```python
from build123d import *

# Parameters (mm, degrees)
SKETCH1_R               = 50.8
BOSS_EXTRUDE1_DEPTH     = 2.54
BOSS_EXTRUDE2_DEPTH     = 10.16
FILLET1_R               = 1.27
CUT_EXTRUDE1_DEPTH      = 113.048264746
CUT_EXTRUDE1_DEPTH_BACK = 113.048264746
SKETCH3_R               = 2.54
SKETCH5_R               = 1.27
CUT_EXTRUDE2_DEPTH      = 73.556912988


# Read off the part's stored shape, not the designer's step: Boss-Extrude2
with BuildPart() as part:
    # Sketch1 → Boss-Extrude1 (new body)
    with BuildSketch(Plane(origin=(0, 0, 0), x_dir=(1, 0, 0), z_dir=(0, 1, 0))):
        with Locations(Location((0, 0, 0), (0, 0, 270))):
            Circle(SKETCH1_R)
    extrude(amount=BOSS_EXTRUDE1_DEPTH)


with BuildPart() as boss_extrude2_tool:
    # Boss-Extrude2 outline → Boss-Extrude2 (new body)
    with BuildSketch(Plane(origin=(0, 2.54, 0), x_dir=(1, 0, 0), z_dir=(0, 1, 0))):
        with BuildLine():
            Line((-5.08, -48.26), (-5.08, -50.545361805))
            add(Edge.make_bspline(
                [(5.08, -50.545361805), (0, -51.054638195), (-5.08, -50.545361805)],
                knots=[0, 0, 0, 1, 1, 1], degree=2))
            Line((5.08, -50.545361805), (5.08, -48.26))
            Line((5.08, -48.26), (-5.08, -48.26))
        make_face()
        with BuildLine():
            Line((5.08, 48.26), (5.08, 50.545361805))
            add(Edge.make_bspline(
                [(-5.08, 50.545361805), (0, 51.054638195), (5.08, 50.545361805)],
                knots=[0, 0, 0, 1, 1, 1], degree=2))
            Line((-5.08, 50.545361805), (-5.08, 48.26))
            Line((-5.08, 48.26), (5.08, 48.26))
        make_face()
    extrude(amount=BOSS_EXTRUDE2_DEPTH)


with BuildPart() as part_1:
    add(part.part)


with BuildPart() as part_2:
    # Boss-Extrude2: joined with boss_extrude2_tool
    add(part_1.part.fuse(boss_extrude2_tool.part, tol=0.00001))

    # Fillet1
    # the kernel refuses this fillet: 1.27 mm, written as the material it adds along each edge
    with BuildSketch(Plane(origin=(-5.08, 2.54, -48.26), x_dir=(0, 0, 1), z_dir=(1, 0, 0)), Plane(origin=(5.08, 2.54, 48.26), x_dir=(0, 0, -1), z_dir=(-1, 0, 0))) as fillet1_piece_1:
        with BuildLine():
            CenterArc((FILLET1_R, -FILLET1_R), FILLET1_R, 90, 90)
            Line((0, -FILLET1_R), (0, 0))
            Line((0, 0), (FILLET1_R, 0))
        make_face()
    extrude(amount=10.16)
    with BuildSketch(Plane(origin=(5.08, 2.54, -48.26), x_dir=(1, 0, 0), z_dir=(0, 0, -1))) as fillet1_piece_2_section:
        with BuildLine():
            CenterArc((FILLET1_R, -FILLET1_R), FILLET1_R, 90, 90)
            Line((0, -FILLET1_R), (0, 0))
            Line((0, 0), (FILLET1_R, 0))
        make_face()
    fillet1_piece_2 = extrude(amount=5.460361805, mode=Mode.PRIVATE)
    fillet1_piece_2 = fillet1_piece_2 & Plane(origin=(0, 2.829642474, 0), x_dir=(0, 0, 1), z_dir=(0, -1, 0)) * Cylinder(50.8, 17, mode=Mode.PRIVATE)
    add(fillet1_piece_2)
    with BuildSketch(Plane(origin=(5.08, 2.54, 53.720361805), x_dir=(1, 0, 0), z_dir=(0, 0, -1))) as fillet1_piece_3_section:
        with BuildLine():
            CenterArc((FILLET1_R, -FILLET1_R), FILLET1_R, 90, 90)
            Line((0, -FILLET1_R), (0, 0))
            Line((0, 0), (FILLET1_R, 0))
        make_face()
    fillet1_piece_3 = extrude(amount=5.460361805, mode=Mode.PRIVATE)
    fillet1_piece_3 = fillet1_piece_3 & Plane(origin=(0, 2.829642639, 0), x_dir=(0, 0, 1), z_dir=(0, -1, 0)) * Cylinder(50.8, 17, mode=Mode.PRIVATE)
    add(fillet1_piece_3)
    with BuildSketch(Plane(origin=(-5.08, 2.54, 48.26), x_dir=(-1, 0, 0), z_dir=(0, 0, 1))) as fillet1_piece_4_section:
        with BuildLine():
            CenterArc((FILLET1_R, -FILLET1_R), FILLET1_R, 90, 90)
            Line((0, -FILLET1_R), (0, 0))
            Line((0, 0), (FILLET1_R, 0))
        make_face()
    fillet1_piece_4 = extrude(amount=5.460361805, mode=Mode.PRIVATE)
    fillet1_piece_4 = fillet1_piece_4 & Plane(origin=(0, 2.829642474, 0), x_dir=(0, 0, 1), z_dir=(0, -1, 0)) * Cylinder(50.8, 17, mode=Mode.PRIVATE)
    add(fillet1_piece_4)
    with BuildSketch(Plane(origin=(-5.08, 2.54, -53.720361805), x_dir=(-1, 0, 0), z_dir=(0, 0, 1))) as fillet1_piece_5_section:
        with BuildLine():
            CenterArc((FILLET1_R, -FILLET1_R), FILLET1_R, 90, 90)
            Line((0, -FILLET1_R), (0, 0))
            Line((0, 0), (FILLET1_R, 0))
        make_face()
    fillet1_piece_5 = extrude(amount=5.460361805, mode=Mode.PRIVATE)
    fillet1_piece_5 = fillet1_piece_5 & Plane(origin=(0, 2.829642639, 0), x_dir=(0, 0, 1), z_dir=(0, -1, 0)) * Cylinder(50.8, 17, mode=Mode.PRIVATE)
    add(fillet1_piece_5)
    with BuildSketch(Plane(origin=(-5.08, 2.54, -53.720361805), x_dir=(-1, 0, 0), z_dir=(0, 0, 1))) as fillet1_piece_6a_section:
        with BuildLine():
            CenterArc((FILLET1_R, -FILLET1_R), FILLET1_R, 90, 90)
            Line((0, -FILLET1_R), (0, 0))
            Line((0, 0), (FILLET1_R, 0))
        make_face()
    fillet1_piece_6a = extrude(amount=8.635361805, mode=Mode.PRIVATE)
    fillet1_piece_6a = split(fillet1_piece_6a, bisect_by=Plane(origin=(-5.367521795, 2.827521795, -48.26), z_dir=(0, 0, 1)), keep=Keep.TOP, mode=Mode.PRIVATE)
    with BuildSketch(Plane(origin=(-8.255, 2.54, -48.26), x_dir=(0, 0, 1), z_dir=(1, 0, 0))) as fillet1_piece_6b_section:
        with BuildLine():
            CenterArc((FILLET1_R, -FILLET1_R), FILLET1_R, 90, 90)
            Line((0, -FILLET1_R), (0, 0))
            Line((0, 0), (FILLET1_R, 0))
        make_face()
    fillet1_piece_6b = extrude(amount=13.335, mode=Mode.PRIVATE)
    fillet1_piece_6b = split(fillet1_piece_6b, bisect_by=Plane(origin=(-5.08, 2.827521795, -47.972478205), z_dir=(-1, 0, 0)), keep=Keep.TOP, mode=Mode.PRIVATE)
    fillet1_piece_6 = fillet1_piece_6a & fillet1_piece_6b
    add(fillet1_piece_6)
    with BuildSketch(Plane(origin=(-5.08, 2.54, -48.26), x_dir=(0, 0, 1), z_dir=(1, 0, 0))) as fillet1_piece_7a_section:
        with BuildLine():
            CenterArc((FILLET1_R, -FILLET1_R), FILLET1_R, 90, 90)
            Line((0, -FILLET1_R), (0, 0))
            Line((0, 0), (FILLET1_R, 0))
        make_face()
    fillet1_piece_7a = extrude(amount=13.335, mode=Mode.PRIVATE)
    fillet1_piece_7a = split(fillet1_piece_7a, bisect_by=Plane(origin=(5.08, 2.827521795, -47.972478205), z_dir=(1, 0, 0)), keep=Keep.TOP, mode=Mode.PRIVATE)
    with BuildSketch(Plane(origin=(5.08, 2.54, -45.085), x_dir=(1, 0, 0), z_dir=(0, 0, -1))) as fillet1_piece_7b_section:
        with BuildLine():
            CenterArc((FILLET1_R, -FILLET1_R), FILLET1_R, 90, 90)
            Line((0, -FILLET1_R), (0, 0))
            Line((0, 0), (FILLET1_R, 0))
        make_face()
    fillet1_piece_7b = extrude(amount=8.635361805, mode=Mode.PRIVATE)
    fillet1_piece_7b = split(fillet1_piece_7b, bisect_by=Plane(origin=(5.367521795, 2.827521795, -48.26), z_dir=(0, 0, 1)), keep=Keep.TOP, mode=Mode.PRIVATE)
    fillet1_piece_7 = fillet1_piece_7a & fillet1_piece_7b
    add(fillet1_piece_7)
    with BuildSketch(Plane(origin=(5.08, 2.54, 53.720361805), x_dir=(1, 0, 0), z_dir=(0, 0, -1))) as fillet1_piece_8a_section:
        with BuildLine():
            CenterArc((FILLET1_R, -FILLET1_R), FILLET1_R, 90, 90)
            Line((0, -FILLET1_R), (0, 0))
            Line((0, 0), (FILLET1_R, 0))
        make_face()
    fillet1_piece_8a = extrude(amount=8.635361805, mode=Mode.PRIVATE)
    fillet1_piece_8a = split(fillet1_piece_8a, bisect_by=Plane(origin=(5.367521795, 2.827521795, 48.26), z_dir=(0, 0, -1)), keep=Keep.TOP, mode=Mode.PRIVATE)
    with BuildSketch(Plane(origin=(8.255, 2.54, 48.26), x_dir=(0, 0, -1), z_dir=(-1, 0, 0))) as fillet1_piece_8b_section:
        with BuildLine():
            CenterArc((FILLET1_R, -FILLET1_R), FILLET1_R, 90, 90)
            Line((0, -FILLET1_R), (0, 0))
            Line((0, 0), (FILLET1_R, 0))
        make_face()
    fillet1_piece_8b = extrude(amount=13.335, mode=Mode.PRIVATE)
    fillet1_piece_8b = split(fillet1_piece_8b, bisect_by=Plane(origin=(5.08, 2.827521795, 47.972478205), z_dir=(1, 0, 0)), keep=Keep.TOP, mode=Mode.PRIVATE)
    fillet1_piece_8 = fillet1_piece_8a & fillet1_piece_8b
    add(fillet1_piece_8)
    with BuildSketch(Plane(origin=(5.08, 2.54, 48.26), x_dir=(0, 0, -1), z_dir=(-1, 0, 0))) as fillet1_piece_9a_section:
        with BuildLine():
            CenterArc((FILLET1_R, -FILLET1_R), FILLET1_R, 90, 90)
            Line((0, -FILLET1_R), (0, 0))
            Line((0, 0), (FILLET1_R, 0))
        make_face()
    fillet1_piece_9a = extrude(amount=13.335, mode=Mode.PRIVATE)
    fillet1_piece_9a = split(fillet1_piece_9a, bisect_by=Plane(origin=(-5.08, 2.827521795, 47.972478205), z_dir=(-1, 0, 0)), keep=Keep.TOP, mode=Mode.PRIVATE)
    with BuildSketch(Plane(origin=(-5.08, 2.54, 45.085), x_dir=(-1, 0, 0), z_dir=(0, 0, 1))) as fillet1_piece_9b_section:
        with BuildLine():
            CenterArc((FILLET1_R, -FILLET1_R), FILLET1_R, 90, 90)
            Line((0, -FILLET1_R), (0, 0))
            Line((0, 0), (FILLET1_R, 0))
        make_face()
    fillet1_piece_9b = extrude(amount=8.635361805, mode=Mode.PRIVATE)
    fillet1_piece_9b = split(fillet1_piece_9b, bisect_by=Plane(origin=(-5.367521795, 2.827521795, 48.26), z_dir=(0, 0, -1)), keep=Keep.TOP, mode=Mode.PRIVATE)
    fillet1_piece_9 = fillet1_piece_9a & fillet1_piece_9b
    add(fillet1_piece_9)

    # Sketch3 → Cut-Extrude1 (cut, two sides: drawn at the far end of the back side and taken through both)
    with BuildSketch(Plane(origin=(0, 0, 48.26), x_dir=(-1, 0, 0), z_dir=(0, 0, -1)).offset(-CUT_EXTRUDE1_DEPTH_BACK)):
        with Locations((0, 7.62)):
            Circle(SKETCH3_R)
    extrude(amount=CUT_EXTRUDE1_DEPTH + CUT_EXTRUDE1_DEPTH_BACK, mode=Mode.SUBTRACT)

    # Sketch5 → Cut-Extrude2 (cut, through all)
    with BuildSketch(Plane(origin=(0, 2.54, 0), x_dir=(1, 0, 0), z_dir=(0, 1, 0))):
        with Locations(Location((-2.54, 43.536503653, 0), (0, 0, 270))):
            Circle(SKETCH5_R)
        with Locations(Location((2.54, 43.536503653, 0), (0, 0, 270))):
            Circle(SKETCH5_R)
        with Locations(Location((2.54, -43.536503653, 0), (0, 0, 90))):
            Circle(SKETCH5_R)
        with Locations(Location((-2.54, -43.536503653, 0), (0, 0, 90))):
            Circle(SKETCH5_R)
    extrude(amount=-CUT_EXTRUDE2_DEPTH, mode=Mode.SUBTRACT)


solid = part_2.part
```
Part model, mm, in its own coordinate system. A direction names the side the tool comes from. Coordinates: 2 decimals unless noted, no trailing zeros. Order: outer loops, then holes, each group sorted by start corner. A loop starts at its lowest first (then second) coordinate and runs counter-clockwise, first axis right, second up. Notation, with made-up numbers: (-34, 38) - (-7, 38) arc R15 cw to (-7, 51) - close; hole circle Ø10 at (29, -28.75). An arc over 180 degrees is marked (long way). Return JSON: item names as keys, results as strings. Group by question number.
Item 1: Cut at A-A (z = 0). List the corners of the cut face in (x, y), plus the area to 3 significant figures.
Item 2: Cut at C-C (x = 14.5). List the corners of the cut face in (y, z).
Item 3: Pull direction X, two halves, no side cores. Call faces 6 (the face through (-1.1, 10.2, 48.26)), 7 (the face through (-5.08, 8, -49)), 8 (the face through (0.55, 5.14, -49.51)): pulls with the +X half, pulls with the -X half, needs draft (parallel to the pull), parting line crosses it, or undercut.
Item 4: Drill centre lines: probe 1 along X at (y, z) = (7.62, 50.1); probe 2 along Y at (x, z) = (9, -29.5); probe 3 along Y at (x, z) = (0, 49.35). Where is each one in solid material? Low to high. Write a range as from..to.
Item 5: Pin check, flat tips, straight feed: pin 1 (1.8 mm diameter, centred on y = 7.5, z = -49, fed in from +X); pin 2 (2.5 mm diameter, centred on x = -1.5, y = 6.5, fed in from -Z); pin 3 (3 mm diameter, centred on y = 3, z = -14.5, fed in from -X); pin 4 (1.5 mm diameter, centred on x = -2.54, z = -43.54, fed in from +Y). Stop position of each tip, or through.
Item 6: Which spindle directions (+Z, -Z, +X, -X, +Y, -Y) get a long thin tool onto all of the face, cutting with end or side? Do faces 1 (the face through (-5.08, 8, 49)), 2 (the face through (5.08, 8, 49)), 3 (the face through (1.1, 10.2, -48.26)), 4 (the face through (2.484, 1.288, 44.805)), 5 (the face through (1, 0, -1)). Say none if no direction does.
Check values:
{
 "1": {"outline": "(-50.8, 0) - (50.8, 0) - (50.8, 2.54) - (-50.8, 2.54) - close", "area": "258 mm2"},
 "2": {"outline": "(0, -48.69) - (2.54, -48.69) - (2.54, 48.69) - (0, 48.69) - close"},
 "3": {"face 6": "needs draft", "face 7": "pulls with the -X half", "face 8": "undercut"},
 "4": {"probe 1": "x = -5.08..-2.54, 2.54..5.08", "probe 2": "y = 0..2.54", "probe 3": "y = 0..5.08, 10.16..12.7"},
 "5": {"pin 1": "stops at x = 5.08", "pin 2": "stops at z = -50.79", "pin 3": "stops at x = -49.09", "pin 4": "passes through"},
 "6": {"face 1": "+Z, -Z, -X, +Y", "face 2": "+Z, -Z, +X, +Y", "face 3": "+X, -X, +Y", "face 4": "+Y, -Y", "face 5": "+Z, -Z, +X, -X, -Y"}
}
